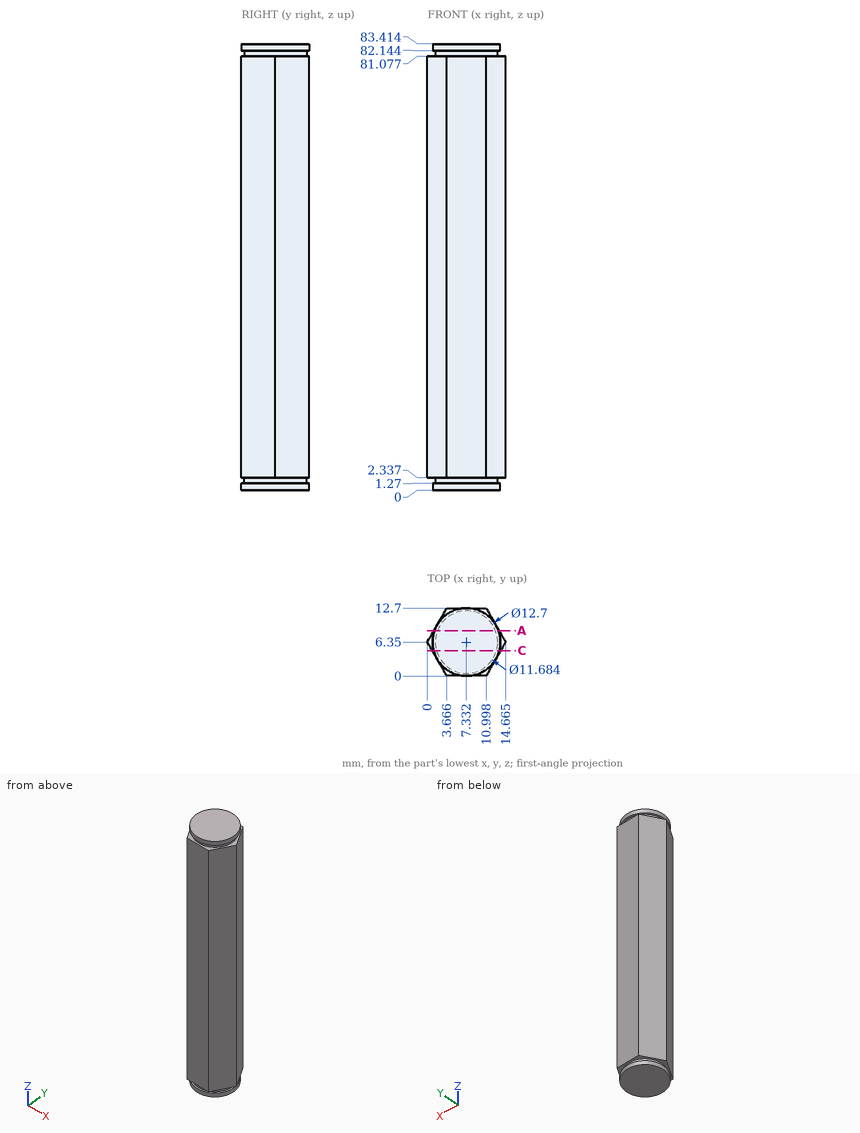
Geometry check sheet. Reference: drawing and pictorial views, mm from the part's lowest x, y, z. Round coordinates to 2 decimals unless told otherwise and drop trailing zeros. Order: outer loops, then holes, each group sorted by start corner. A loop starts at its lowest first (then second) coordinate and runs counter-clockwise, first axis right, second up. Notation, with made-up numbers: (29, 16.5) -> (83, 16.5) arc R18 ccw to (83, 50.5) -> close; hole circle Ø7 at (0.25, -29.75). An arc over 180 degrees is marked (long way). One line per item, written item: value. Start each with the question number.
Q1. Gauge pin test, flat end, axial feed: pin 1 Ø4 at (y, z) = (10, 44) entering from -X. Record the tip position at first contact, or that the pin passes through.
Q2. Cross-section at C-C (y = 4.75). Record the boundary of the cut face in (x, z), and give its area (3 significant figures).
Q3. Cross-section at A-A (y = 8.5). Record the boundary of the cut face in (x, z) (1 decimal), and give its area (3 significant figures).
Q4. Thickness scan on line 1 (Z direction, x = 7.25, y = 12.25); line 2 (X direction, y = 2.75, z = 46) (1 decimal); line 3 (X direction, y = 5.5, z = 44) (1 decimal). Record the ranges inside material, lowest first.
Completed:
1. pin 1: stops at x = 0.95
2. outline: (0.92, 2.34) -> (1.71, 2.34) -> (1.71, 1.27) -> (1.19, 1.27) -> (1.19, 0) -> (13.48, 0) -> (13.48, 1.27) -> (12.95, 1.27) -> (12.95, 2.34) -> (13.74, 2.34) -> (13.74, 81.08) -> (12.95, 81.08) -> (12.95, 82.14) -> (13.48, 82.14) -> (13.48, 83.41) -> (1.19, 83.41) -> (1.19, 82.14) -> (1.71, 82.14) -> (1.71, 81.08) -> (0.92, 81.08) -> close
2. area: 1,060 mm²
3. outline: (1.2, 2.3) -> (1.9, 2.3) -> (1.9, 1.3) -> (1.4, 1.3) -> (1.4, 0) -> (13.3, 0) -> (13.3, 1.3) -> (12.8, 1.3) -> (12.8, 2.3) -> (13.4, 2.3) -> (13.4, 81.1) -> (12.8, 81.1) -> (12.8, 82.1) -> (13.3, 82.1) -> (13.3, 83.4) -> (1.4, 83.4) -> (1.4, 82.1) -> (1.9, 82.1) -> (1.9, 81.1) -> (1.2, 81.1) -> close
3. area: 1,010 mm²
4. line 1: z = 0 to 1.27, 2.34 to 81.08, 82.14 to 83.41
4. line 2: x = 2.1 to 12.6
4. line 3: x = 0.5 to 14.2
